Verification items for the finished model (mm, model axes). Face numbers are marked on the shaded views. A direction names the side the tool comes from. Give positions to 0.01 mm unless a question says otherwise; leave off trailing zeros. Loops run counter-clockwise (first coordinate to the right, second up) from the corner with the lowest first, then second, coordinate; pieces in that order, holes last. Notation, with made-up numbers: M 87.25,37.25 L 97.25,37.25 A24 ccw 97.25,72.25 Z; hole C -7.75,22.5 d2. An arc over 180 degrees is marked long. Put each result on its own line as item: value. Start each with the question number.
from build123d import *

# Parameters (mm, degrees)
SKETCH1_W           = 150
SKETCH1_H           = 100
SKETCH1_R           = 10
BOSS_EXTRUDE1_DEPTH = 15
SKETCH2_R           = 10
BOSS_EXTRUDE2_DEPTH = 7.5
BOSS_EXTRUDE3_DEPTH = 7.5


with BuildPart() as part:
    # Sketch1 → Boss-Extrude1 (new body)
    with BuildSketch(Plane(origin=(0, 0, 0), x_dir=(1, 0, 0), z_dir=(0, 1, 0))):
        Rectangle(SKETCH1_W, SKETCH1_H)
        with Locations(Location((-45, 30, 0), (0, 0, 270))):
            Circle(SKETCH1_R, mode=Mode.SUBTRACT)
        with Locations(Location((45, 30, 0), (0, 0, 270))):
            Circle(SKETCH1_R, mode=Mode.SUBTRACT)
        with Locations(Location((45, -30, 0), (0, 0, 270))):
            Circle(SKETCH1_R, mode=Mode.SUBTRACT)
        with Locations(Location((-45, -30, 0), (0, 0, 270))):
            Circle(SKETCH1_R, mode=Mode.SUBTRACT)
    extrude(amount=BOSS_EXTRUDE1_DEPTH)

    # Sketch2 → Boss-Extrude2 (add, symmetric)
    with BuildSketch(Plane.XY):
        with BuildLine():
            Line((75, 15), (-75, 15))
            Line((-75, 15), (-144.282032303, 55))
            ThreePointArc((-144.282032303, 55), (-154.13052805, 87.855309915), (-121.911493446, 99.61958071))
            Line((-121.911493446, 99.61958071), (75, 15))
        make_face()
        with Locations((-131.782032303, 76.650635095)):
            Circle(SKETCH2_R, mode=Mode.SUBTRACT)
    extrude(amount=BOSS_EXTRUDE2_DEPTH, both=True)

    # Sketch3 → Boss-Extrude3 (add, symmetric)
    with BuildSketch(Plane(origin=(0, 0, 0), x_dir=(0, 0, -1), z_dir=(1, 0, 0))):
        Polygon((-7.5, 35), (-7.5, 15), (-50, 15), align=None)
        Polygon((50, 15), (7.5, 35), (7.5, 15), align=None)
    extrude(amount=BOSS_EXTRUDE3_DEPTH, both=True)


solid = part.part
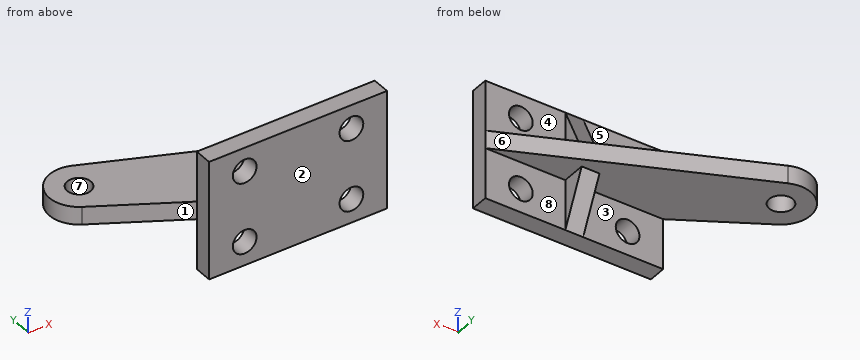
Q1. Release check for a two-part mould opening along X. For the marked faces 6, 7 and 8 record: pulls with the +X half, pulls with the -X half, needs draft (parallel to the pull), parting line crosses it, or undercut.
Q2. Cross-section at A-A, the plane z = -34.5. Record the boundary of the cut face in (x, y), then the cut area to 3 significant figures.
Q3. Cross-section at B-B, the plane x = -51. Record the boundary of the cut face in (y, z), then the cut area to 3 significant figures.
Q4. Scan lines: L1, parallel to Y at x = 11, z = -38.5; L2, parallel to X at y = 84, z = 0; L3, parallel to X at y = 75.5, z = -7. Record each from-to range of solid material in increasing order.
Q5. Cross-section at C-C, the plane z = 4.5. Record the boundary of the cut face in (x, y).
Q6. Go/stop test with flat-tipped pins: pin 1 (13 mm diameter, centred on x = 58, z = -21, fed in from +Y); pin 2 (10 mm diameter, centred on y = 24.5, z = -27, fed in from -X); pin 3 (6 mm diameter, centred on y = 24.5, z = -36, fed in from +X); pin 4 (12 mm diameter, centred on x = -5.5, z = -24.5, fed in from -Y). Record where each tip stops, or that it passes through.
Q7. Cross-section at D-D, the plane z = -10. Record the boundary of the cut face in (x, y), then the cut area to 3 significant figures.
Q8. Set-up check for the marked faces 1, 2, 3, 4 and 5: record each of +Z, -Z, +X, -X, +Y, -Y from which the full face is reachable in a straight line by a thin tool's end or side.
Ans:
1. face 6: pulls with the +X half
1. face 7: undercut
1. face 8: needs draft
2. outline: M -75,0 L -53.93,0 L -53.93,15 L -75,15 Z; M -36.07,0 L 36.07,0 L 36.07,15 L 7.5,15 L 7.5,22.29 L -7.5,22.29 L -7.5,15 L -36.07,15 Z; M 53.93,0 L 75,0 L 75,15 L 53.93,15 Z
2. area: 1,820 mm^2
3. outline: M 0,-50 L 15,-50 L 15,-38 L 0,-38 Z; M 0,-22 L 15,-22 L 15,-7.5 L 69.15,-7.5 L 69.15,7.5 L 15,7.5 L 15,22 L 0,22 Z; M 0,38 L 15,38 L 15,50 L 0,50 Z
3. area: 1,830 mm^2
4. L1: y = 0 to 15
4. L2: x = -155.68 to -138.56, -125 to -85.56
4. L3: x = -156.76 to -141.72, -121.85 to -65.78
5. outline: M -144.28,55 L -75,15 L -75,0 L 75,0 L 75,15 L -121.91,99.62 A25 ccw Z; hole C -131.78,76.65 d20
6. pin 1: stops at y = 15
6. pin 2: stops at x = -7.5
6. pin 3: stops at x = 7.5
6. pin 4: stops at y = 0
7. outline: M -75,0 L 75,0 L 75,15 L 7.5,15 L 7.5,33.82 L -7.5,33.82 L -7.5,15 L -75,15 Z
7. area: 2,530 mm^2
8. face 1: +Z, -Z, -X, -Y
8. face 2: +Z, -Z, +X, -X, -Y
8. face 3: -Z, -X, +Y
8. face 4: +Z, +X, +Y
8. face 5: +Z, -X, +Y
